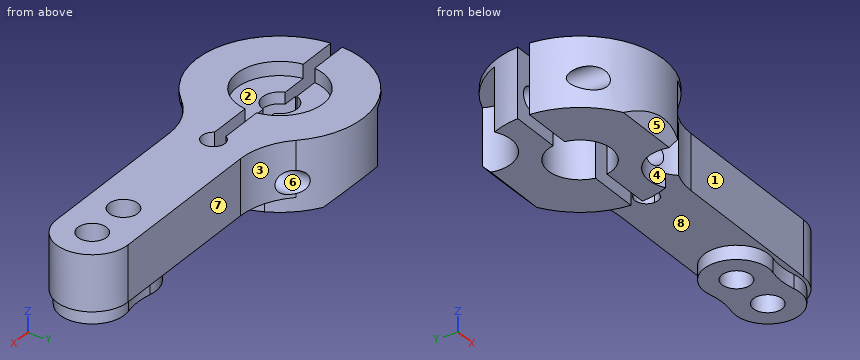
from build123d import *

# Parameters (mm, degrees)
SKETCH_1_R               = 1.25
EXTRUDE_1_DEPTH          = 6
CUT_EXTRUDE_1_DEPTH      = 1.2
SKETCH_1_4_R             = 2.75
CUT_EXTRUDE_2_DEPTH      = 3.8
CUT_EXTRUDE_START        = 6
SKETCH_1_5_R             = 3.75
CUT_EXTRUDE_3_DEPTH      = 1.2
FILLET_1_R               = 6
SKETCH_2_R               = 3
CUT_EXTRUDE_4_DEPTH      = 5.5
SKETCH_3_R               = 1
CUT_EXTRUDE_5_DEPTH      = 8.25
CUT_EXTRUDE_5_DEPTH_BACK = 8.25
CUT_EXTRUDE_6_DEPTH      = 28.1
CUT_EXTRUDE_6_DEPTH_BACK = 8.232738171


with BuildPart() as part:
    # Эскиз1 → Бобышка-Вытянуть1 (new body)
    with BuildSketch(Plane.XY):
        with BuildLine():
            ThreePointArc((24, -3.1), (27.1, 0), (24, 3.1))
            Line((24, 3.1), (6.553815682, 3.1))
            ThreePointArc((6.553815682, 3.1), (7.014789099, 1.831729757), (7.232738071, 0.5))
            Line((7.232738071, 0.5), (7.633974596, 0.5))
            ThreePointArc((7.633974596, 0.5), (8.758819045, 0.965925826), (9.5, 0))
            ThreePointArc((9.5, 0), (8.758819045, -0.965925826), (7.633974596, -0.5))
            Line((7.633974596, -0.5), (7.232738071, -0.5))
            ThreePointArc((7.232738071, -0.5), (7.014789099, -1.831729757), (6.553815682, -3.1))
            Line((6.553815682, -3.1), (24, -3.1))
        make_face()
        with BuildLine():
            ThreePointArc((23.363636364, 2.726727218), (26.8, 0), (23.363636364, -2.726727218))
            ThreePointArc((23.363636364, -2.726727218), (22, -2.569714114), (20.636363636, -2.726727218))
            ThreePointArc((20.636363636, -2.726727218), (17.2, 0), (20.636363636, 2.726727218))
            ThreePointArc((20.636363636, 2.726727218), (22, 2.569714114), (23.363636364, 2.726727218))
        make_face(mode=Mode.SUBTRACT)
        with BuildLine():
            ThreePointArc((20.636363636, 2.726727218), (22, 2.569714114), (23.363636364, 2.726727218))
            ThreePointArc((23.363636364, 2.726727218), (26.8, 0), (23.363636364, -2.726727218))
            ThreePointArc((23.363636364, -2.726727218), (22, -2.569714114), (20.636363636, -2.726727218))
            ThreePointArc((20.636363636, -2.726727218), (17.2, 0), (20.636363636, 2.726727218))
        make_face()
        with Locations((20, 0)):
            Circle(SKETCH_1_R, mode=Mode.SUBTRACT)
        with Locations((24, 0)):
            Circle(SKETCH_1_R, mode=Mode.SUBTRACT)
        with BuildLine():
            ThreePointArc((7.232738071, 0.5), (7.014789099, 1.831729757), (6.553815682, 3.1))
            ThreePointArc((6.553815682, 3.1), (-1.343589931, 7.124413386), (-7.232738071, 0.5))
            Line((-7.232738071, 0.5), (-3.716517187, 0.5))
            ThreePointArc((-3.716517187, 0.5), (0, 3.75), (3.716517187, 0.5))
            Line((3.716517187, 0.5), (7.232738071, 0.5))
        make_face()
        with BuildLine():
            ThreePointArc((3.716517187, 0.5), (0, 3.75), (-3.716517187, 0.5))
            Line((-3.716517187, 0.5), (-2.704163457, 0.5))
            ThreePointArc((-2.704163457, 0.5), (0, 2.75), (2.704163457, 0.5))
            Line((2.704163457, 0.5), (3.716517187, 0.5))
        make_face()
        with BuildLine():
            ThreePointArc((2.704163457, 0.5), (0, 2.75), (-2.704163457, 0.5))
            Line((-2.704163457, 0.5), (-1.414213562, 0.5))
            ThreePointArc((-1.414213562, 0.5), (0, 1.5), (1.414213562, 0.5))
            Line((1.414213562, 0.5), (2.704163457, 0.5))
        make_face()
        with BuildLine():
            ThreePointArc((-7.232738071, -0.5), (-1.343589931, -7.124413386), (6.553815682, -3.1))
            ThreePointArc((6.553815682, -3.1), (7.014789099, -1.831729757), (7.232738071, -0.5))
            Line((7.232738071, -0.5), (3.716517187, -0.5))
            ThreePointArc((3.716517187, -0.5), (0, -3.75), (-3.716517187, -0.5))
            Line((-3.716517187, -0.5), (-7.232738071, -0.5))
        make_face()
        with BuildLine():
            Line((-2.704163457, -0.5), (-3.716517187, -0.5))
            ThreePointArc((-3.716517187, -0.5), (0, -3.75), (3.716517187, -0.5))
            Line((3.716517187, -0.5), (2.704163457, -0.5))
            ThreePointArc((2.704163457, -0.5), (0, -2.75), (-2.704163457, -0.5))
        make_face()
        with BuildLine():
            Line((-1.414213562, -0.5), (-2.704163457, -0.5))
            ThreePointArc((-2.704163457, -0.5), (0, -2.75), (2.704163457, -0.5))
            Line((2.704163457, -0.5), (1.414213562, -0.5))
            ThreePointArc((1.414213562, -0.5), (0, -1.5), (-1.414213562, -0.5))
        make_face()
    extrude(amount=EXTRUDE_1_DEPTH)

    # Эскиз1<3> → Вырез-Вытянуть1 (cut)
    with BuildSketch(Plane.XY):
        with BuildLine():
            ThreePointArc((24, -3.1), (27.1, 0), (24, 3.1))
            Line((24, 3.1), (6.553815682, 3.1))
            ThreePointArc((6.553815682, 3.1), (7.014789099, 1.831729757), (7.232738071, 0.5))
            Line((7.232738071, 0.5), (7.633974596, 0.5))
            ThreePointArc((7.633974596, 0.5), (8.758819045, 0.965925826), (9.5, 0))
            ThreePointArc((9.5, 0), (8.758819045, -0.965925826), (7.633974596, -0.5))
            Line((7.633974596, -0.5), (7.232738071, -0.5))
            ThreePointArc((7.232738071, -0.5), (7.014789099, -1.831729757), (6.553815682, -3.1))
            Line((6.553815682, -3.1), (24, -3.1))
        make_face()
        with BuildLine():
            ThreePointArc((23.363636364, 2.726727218), (26.8, 0), (23.363636364, -2.726727218))
            ThreePointArc((23.363636364, -2.726727218), (22, -2.569714114), (20.636363636, -2.726727218))
            ThreePointArc((20.636363636, -2.726727218), (17.2, 0), (20.636363636, 2.726727218))
            ThreePointArc((20.636363636, 2.726727218), (22, 2.569714114), (23.363636364, 2.726727218))
        make_face(mode=Mode.SUBTRACT)
    extrude(amount=CUT_EXTRUDE_1_DEPTH, mode=Mode.SUBTRACT)

    # Эскиз1<4> → Вырез-Вытянуть2 (cut)
    with BuildSketch(Plane.XY):
        Circle(SKETCH_1_4_R)
    extrude(amount=CUT_EXTRUDE_2_DEPTH, mode=Mode.SUBTRACT)

    # Эскиз1<5> → Вырез-Вытянуть3 (cut)
    with BuildSketch(Plane.XY.offset(CUT_EXTRUDE_START)):
        Circle(SKETCH_1_5_R)
    extrude(amount=-CUT_EXTRUDE_3_DEPTH, mode=Mode.SUBTRACT)

    # Скругление1
    fillet_1_edges = [part.edges().sort_by_distance(p)[0] for p in [
        (6.553815682, 3.1, 3.6),
        (6.553815682, -3.1, 3.6),
    ]]
    fillet(fillet_1_edges, radius=FILLET_1_R)

    # Эскиз2 → Вырез-Вытянуть4 (cut)
    with BuildSketch(Plane.XY):
        with Locations((5.099019514, -5.5)):
            Circle(SKETCH_2_R)
        with Locations((-5.099019514, 5.5)):
            Circle(SKETCH_2_R)
    extrude(amount=CUT_EXTRUDE_4_DEPTH, mode=Mode.SUBTRACT)

    # Эскиз3 → Вырез-Вытянуть5 (cut, two sides)
    with BuildSketch(Plane(origin=(0, 0, 0), x_dir=(1, 0, 0), z_dir=(0, 1, 0))) as cut_extrude_5_sk:
        with Locations((5.5, -2.5)):
            Circle(SKETCH_3_R)
        with Locations((-5.5, -2.5)):
            Circle(SKETCH_3_R)
    extrude(amount=CUT_EXTRUDE_5_DEPTH, mode=Mode.SUBTRACT)
    extrude(cut_extrude_5_sk.sketch, amount=-CUT_EXTRUDE_5_DEPTH_BACK, mode=Mode.SUBTRACT)

    # Эскиз4 → Вырез-Вытянуть6 (cut, two sides)
    with BuildSketch(Plane(origin=(0, 0, 0), x_dir=(0, 0, -1), z_dir=(1, 0, 0))) as cut_extrude_6_sk:
        Polygon((0, -6.25), (-1, -7.25), (0, -7.25), align=None)
        Polygon((0, 7.25), (0, 6.25), (-1, 7.25), align=None)
    extrude(amount=CUT_EXTRUDE_6_DEPTH, mode=Mode.SUBTRACT)
    extrude(cut_extrude_6_sk.sketch, amount=-CUT_EXTRUDE_6_DEPTH_BACK, mode=Mode.SUBTRACT)


solid = part.part
Check sheet for the modelled part. Datum: model origin and axes. Units: mm. Face numbers are marked on the shaded views. A direction names the side the tool comes from. Coordinates: 2 decimals unless noted, no trailing zeros. Write each loop counter-clockwise with the first axis right and the second up, starting at its lowest first coordinate (ties: lowest second). Pieces come first, ordered by that corner, then holes.
Item 1: Cross-section at B-B on x = -5.5. Record the boundary of the cut face in (y, z), then the cut area to 3 significant figures.
Numbers:
outline: (-4.72, 0) - (-0.5, 0) - (-0.5, 1.5) - (-4.72, 1.5) - close; (-4.72, 3.5) - (-0.5, 3.5) - (-0.5, 6) - (-4.72, 6) - close; (0.5, 0) - (2.53, 0) - (2.53, 1.5) - (0.5, 1.5) - close; (0.5, 3.5) - (2.53, 3.5) - (2.53, 5.5) - (4.72, 5.5) - (4.72, 6) - (0.5, 6) - close
area: 26.1 mm2
Item 2: Cross-section at D-D on x = 12.5. Record the boundary of the cut face in (y, z), then the cut area to 3 significant figures.
Numbers:
outline: (-3.1, 1.2) - (3.1, 1.2) - (3.1, 6) - (-3.1, 6) - close
area: 29.8 mm2
Item 3: Cross-section at C-C on z = 2. Count the separate pieces of the cut face and the enclosed holes in it, then the cut area to 3 significant figures.
Numbers:
separate pieces: 5
enclosed holes: 2
area: 196 mm2
Item 4: Mould release check, pull along Z, two halves, no side actions. Record for the marked faces 6, 7 and 8: released by +Z, released by -Z, zero draft, split by the parting line, or undercut.
Numbers:
face 6: undercut
face 7: zero draft
face 8: released by -Z
Item 5: Access from +Z, -Z, +X, -X, +Y, -Y to the whole of each face (thin tool, end or side, straight path). Record for the marked faces 1, 2, 3, 4 and 5.
Numbers:
face 1: +Z, -Z, +X, -Y
face 2: +Z
face 3: +Z, -Z, +X, +Y
face 4: -Z
face 5: -Z, +X, -X, -Y
Item 6: Depth check by flat-ended pin: pin 1 Ø1.5 at (x, z) = (7.5, 4) entering from +Y; pin 2 Ø3.5 at (x, y) = (5.5, -5.5) entering from -Z; pin 3 Ø1.8 at (x, z) = (-5.5, 2.5) entering from +Y; pin 4 Ø3.5 at (x, y) = (-1, -2) entering from +Z. Enter the tip coordinate at first touch or a pass-through.
Numbers:
pin 1: stops at y = 3.84
pin 2: stops at z = 5.5
pin 3: passes through
pin 4: stops at z = 6
Item 7: Scan lines: probe 1 along Y at (x, z) = (24, 3.4); probe 2 along Z at (x, y) = (-5.5, 1.15); probe 3 along Y at (x, z) = (0, 4). Record each from-to range of solid material in increasing order.
Numbers:
probe 1: y = -3.1 to -1.25, 1.25 to 3.1
probe 2: z = 0 to 1.5, 3.5 to 6
probe 3: y = -7.25 to -1.5, 1.5 to 7.25
Item 8: Cross-section at A-A on x = 20. Record the boundary of the cut face in (y, z), then the cut area to 3 significant figures.
Numbers:
outline: (-3.1, 1.2) - (-2.8, 1.2) - (-2.8, 0) - (-1.25, 0) - (-1.25, 6) - (-3.1, 6) - close; (1.25, 0) - (2.8, 0) - (2.8, 1.2) - (3.1, 1.2) - (3.1, 6) - (1.25, 6) - close
area: 21.5 mm2
